Source: CAD feature listing. Evaluate the final solid. Frame: model axes, mm. Round coordinates to 2 decimals unless told otherwise and drop trailing zeros. Loops run counter-clockwise (first coordinate to the right, second up) from the corner with the lowest first, then second, coordinate; pieces in that order, holes last. Notation, with made-up numbers: (77, 84) -> (125, 84) arc R15 cw to (125, 112) -> close; hole circle Ø1 at (5, 3.25). An arc over 180 degrees is marked (long way). Put each result on its own line as item: value. Start each with the question number.
1. Cut plane B-B (y = 80). Return the cut outline in (x, z).
2. Material intervals for L1, parallel to Y at x = -30, z = 1.9; L2, parallel to X at y = 22, z = 1.55; L3, parallel to Y at x = -27, z = 3.9, sorted ascending.
3. Cut plane A-A (x = -30). Return the cut outline in (y, z).
4. Cut plane C-C (z = 1.15). State how many separate pieces and enclosed holes the cut face has, then the cut area to 3 significant figures.
5. Contact query for flat-ended pins moving along their axis: pin 1 (2.5 mm diameter, centred on x = -98, z = 3.5, fed in from -Y); pin 2 (6 mm diameter, centred on x = -30, y = 20, fed in from +Z); pin 3 (3 mm diameter, centred on y = 84.5, z = 0.5, fed in from -X); pin 4 (1.5 mm diameter, centred on y = 68, z = 1.5, fed in from +X). Output: stop coordinate, or through.
```python
from build123d import *

# Parameters (mm, degrees)
SKETCH_1_W          = 200
SKETCH_1_H          = 140
SKETCH_1_R          = 3.25
EXTRUDE_1_DEPTH     = 5
FILLET_1_R          = 20
SKETCH_3_W          = 5
SKETCH_3_H          = 25
SKETCH_3_H_2        = 22.807543944
CUT_EXTRUDE_1_DEPTH = 39
SKETCH_4_R          = 1.55
CUT_EXTRUDE_2_DEPTH = 10


with BuildPart() as part:
    # 草图1 → 凸台-拉伸1 (new body)
    with BuildSketch(Plane.XY):
        with Locations((0, 50)):
            Rectangle(SKETCH_1_W, SKETCH_1_H)
        with Locations((30, 80)):
            Circle(SKETCH_1_R, mode=Mode.SUBTRACT)
        with Locations(Location((30, 20, 0), (0, 0, 180))):
            Circle(SKETCH_1_R, mode=Mode.SUBTRACT)
        with Locations(Location((-30, 80, 0), (0, 0, 180))):
            Circle(SKETCH_1_R, mode=Mode.SUBTRACT)
        with Locations((-30, 20)):
            Circle(SKETCH_1_R, mode=Mode.SUBTRACT)
    extrude(amount=EXTRUDE_1_DEPTH)

    # 圆角1
    fillet_1_edges = [part.edges().sort_by_distance(p)[0] for p in [
        (-100, 120, 2.5),
        (-100, -20, 2.5),
        (100, -20, 2.5),
        (100, 120, 2.5),
    ]]
    fillet(fillet_1_edges, radius=FILLET_1_R)

    # 草图3 → 切除-拉伸1 (cut)
    with BuildSketch(Plane.XY.offset(5)):
        with Locations((97.5, 75)):
            Rectangle(SKETCH_3_W, SKETCH_3_H)
        with Locations((97.5, 25)):
            Rectangle(SKETCH_3_W, SKETCH_3_H)
        with Locations((-97.5, 25)):
            Rectangle(SKETCH_3_W, SKETCH_3_H)
        with Locations((-97.5, 75)):
            Rectangle(SKETCH_3_W, SKETCH_3_H)
        with Locations((-97.5, -11.403771972)):
            Rectangle(SKETCH_3_W, SKETCH_3_H_2)
        with Locations((97.5, -11.403771972)):
            Rectangle(SKETCH_3_W, SKETCH_3_H_2)
        with Locations((-97.5, 111.403771972)):
            Rectangle(SKETCH_3_W, SKETCH_3_H_2)
        with Locations((97.5, 111.403771972)):
            Rectangle(SKETCH_3_W, SKETCH_3_H_2)
    extrude(amount=-CUT_EXTRUDE_1_DEPTH, mode=Mode.SUBTRACT)

    # 草图4 → 切除-拉伸2 (cut)
    with BuildSketch(Plane.XY.offset(5)):
        with Locations((95, 85.95)):
            Circle(SKETCH_4_R)
        with Locations((95, 64.05)):
            Circle(SKETCH_4_R)
        with Locations((95, 35.95)):
            Circle(SKETCH_4_R)
        with Locations((95, 14.05)):
            Circle(SKETCH_4_R)
        with Locations((-95, 14.05)):
            Circle(SKETCH_4_R)
        with Locations((-95, 35.95)):
            Circle(SKETCH_4_R)
        with Locations((-95, 64.05)):
            Circle(SKETCH_4_R)
        with Locations((-95, 85.95)):
            Circle(SKETCH_4_R)
        with Locations((95, -1.55)):
            Circle(SKETCH_4_R)
        with Locations((-95, -1.55)):
            Circle(SKETCH_4_R)
        with Locations((95, 101.55)):
            Circle(SKETCH_4_R)
        with Locations((-95, 101.55)):
            Circle(SKETCH_4_R)
    extrude(amount=-CUT_EXTRUDE_2_DEPTH, mode=Mode.SUBTRACT)


solid = part.part
```
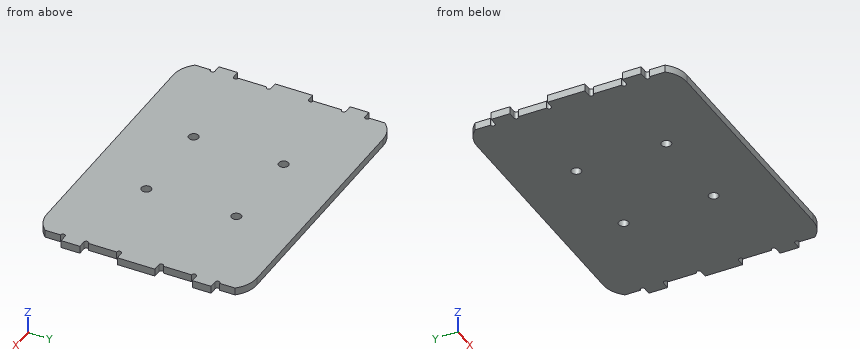
Solution:
1. outline: (-95, 0) -> (-33.25, 0) -> (-33.25, 5) -> (-95, 5) -> close; (-26.75, 0) -> (26.75, 0) -> (26.75, 5) -> (-26.75, 5) -> close; (33.25, 0) -> (95, 0) -> (95, 5) -> (33.25, 5) -> close
2. L1: y = -20 to 16.75, 23.25 to 76.75, 83.25 to 120
2. L2: x = -95 to -32.56, -27.44 to 27.44, 32.56 to 95
2. L3: y = -20 to 18.75, 21.25 to 78.75, 81.25 to 120
3. outline: (-20, 0) -> (16.75, 0) -> (16.75, 5) -> (-20, 5) -> close; (23.25, 0) -> (76.75, 0) -> (76.75, 5) -> (23.25, 5) -> close; (83.25, 0) -> (120, 0) -> (120, 5) -> (83.25, 5) -> close
4. separate pieces: 1
4. enclosed holes: 4
4. area: 26,800 mm^2
5. pin 1: stops at y = 0
5. pin 2: passes through
5. pin 3: stops at x = -95
5. pin 4: stops at x = 95
